```python
from build123d import *

# Parameters (mm, degrees)
SKETCH1_R           = 1.05
BOSS_EXTRUDE1_DEPTH = 1.5
FILLET1_R           = 1.5
SKETCH2_R           = 1.05
SKETCH2_W           = 4
SKETCH2_H           = 16
BOSS_EXTRUDE2_DEPTH = 1.5
SKETCH4_R           = 1.25
CUT_EXTRUDE2_DEPTH  = 160.067595694
CUT_EXTRUDE4_DEPTH  = 160.067595694
FILLET3_R           = 1
FILLET4_R           = 1.5
SKETCH6_W           = 140
SKETCH6_H           = 59.5
CUT_EXTRUDE5_DEPTH  = 10


with BuildPart() as part:
    # Sketch1 → Boss-Extrude1 (new body)
    with BuildSketch(Plane(origin=(0, 0, 0), x_dir=(0, 0, -1), z_dir=(1, 0, 0))):
        Polygon((0, 0), (0, 75.5), (21.5, 75.5), (40, 0), (35.881667859, 0), (29.755840045, 25), (4, 25), (4, 0), align=None)
        with Locations((5.5, 72.5)):
            Circle(SKETCH1_R, mode=Mode.SUBTRACT)
        with Locations((18.5, 72.5)):
            Circle(SKETCH1_R, mode=Mode.SUBTRACT)
        Polygon((4, 69.5), (18.851866535, 69.5), (4, 29), align=None, mode=Mode.SUBTRACT)
        Polygon((8.260475549, 29), (20.558388216, 62.535546651), (28.775707595, 29), align=None, mode=Mode.SUBTRACT)
    extrude(amount=BOSS_EXTRUDE1_DEPTH)

    # Fillet1
    fillet1_edges = [part.edges().sort_by_distance(p)[0] for p in [
        (0.75, 75.5, -21.5),
        (0.75, 25, -29.755840045),
        (0.75, 25, -4),
        (0.75, 69.5, -4),
        (0.75, 29, -4),
        (0.75, 69.5, -18.851866535),
        (0.75, 29, -8.260475549),
        (0.75, 29, -28.775707595),
        (0.75, 62.535546651, -20.558388216),
    ]]
    fillet(fillet1_edges, radius=FILLET1_R)

    # Sketch2 → Boss-Extrude2 (add)
    # profile 1 of 5: a face of its own
    with BuildSketch(Plane(origin=(1.5, 0, 0), x_dir=(0, 0, -1), z_dir=(1, 0, 0))):
        Polygon((70, 0), (70, 16), (36.079470199, 16), (40, 0), align=None)
    # profile 2 of 5: a face of its own
    with BuildSketch(Plane(origin=(1.5, 0, 0), x_dir=(0, 0, -1), z_dir=(1, 0, 0))):
        with BuildLine():
            Line((103.920529801, 16), (70, 16))
            Line((70, 16), (70, 0))
            Line((70, 0), (140, 0))
            Line((140, 0), (140, 16))
            Line((140, 16), (140, 75.5))
            Line((140, 75.5), (119.676824884, 75.5))
            ThreePointArc((119.676824884, 75.5), (118.750942408, 75.180144754), (118.219924421, 74.356988855))
            Line((118.219924421, 74.356988855), (103.920529801, 16))
        make_face()
        with BuildLine():
            Line((108.038861942, 16), (109.964084377, 23.856988855))
            ThreePointArc((109.964084377, 23.856988855), (110.495102363, 24.680144754), (111.420984839, 25))
            Line((111.420984839, 25), (134.5, 25))
            ThreePointArc((134.5, 25), (135.560660172, 24.560660172), (136, 23.5))
            Line((136, 23.5), (136, 16))
            Line((136, 16), (108.038861942, 16))
        make_face(mode=Mode.SUBTRACT)
        with BuildLine():
            ThreePointArc((131.000070484, 31.016439186), (130.821545012, 29.641122471), (129.591776989, 29))
            Line((129.591776989, 29), (113.136216627, 29))
            ThreePointArc((113.136216627, 29), (111.956071873, 29.574117524), (111.679316165, 30.856988855))
            Line((111.679316165, 30.856988855), (118.270545293, 57.756329353))
            ThreePointArc((118.270545293, 57.756329353), (119.644098522, 58.897023121), (121.135739251, 57.915779684))
            Line((121.135739251, 57.915779684), (131.000070484, 31.016439186))
        make_face(mode=Mode.SUBTRACT)
        with BuildLine():
            ThreePointArc((121.887587432, 67.483560814), (122.066112904, 68.858877529), (123.295880927, 69.5))
            Line((123.295880927, 69.5), (134.5, 69.5))
            ThreePointArc((134.5, 69.5), (135.560660172, 69.060660172), (136, 68))
            Line((136, 68), (136, 37.447151885))
            ThreePointArc((136, 37.447151885), (134.762259183, 35.970256452), (133.091706505, 36.930712699))
            Line((133.091706505, 36.930712699), (121.887587432, 67.483560814))
        make_face(mode=Mode.SUBTRACT)
        with Locations((121.5, 72.5)):
            Circle(SKETCH2_R, mode=Mode.SUBTRACT)
        with Locations((134.5, 72.5)):
            Circle(SKETCH2_R, mode=Mode.SUBTRACT)
    # profile 3 of 5: a face of its own
    with BuildSketch(Plane(origin=(1.5, 0, 0), x_dir=(0, 0, -1), z_dir=(1, 0, 0))):
        Polygon((35.881667859, 0), (31.961138058, 16), (4, 16), (4, 0), align=None)
    # profile 4 of 5: a face of its own
    with BuildSketch(Plane(origin=(1.5, 0, 0), x_dir=(0, 0, -1), z_dir=(1, 0, 0))):
        Polygon((40, 0), (36.079470199, 16), (31.961138058, 16), (35.881667859, 0), align=None)
    # profile 5 of 5: a face of its own
    with BuildSketch(Plane(origin=(1.5, 0, 0), x_dir=(0, 0, -1), z_dir=(1, 0, 0))):
        with Locations((2, 8)):
            Rectangle(SKETCH2_W, SKETCH2_H)
    extrude(amount=-BOSS_EXTRUDE2_DEPTH)

    # Sketch4 → Cut-Extrude2 (cut, through all)
    with BuildSketch(Plane(origin=(1.5, 0, 0), x_dir=(0, 0, -1), z_dir=(1, 0, 0))):
        with Locations((6.1, 8)):
            Circle(SKETCH4_R)
        with Locations((17.1, 8)):
            Circle(SKETCH4_R)
        with Locations(Location((122.9, 8, 0), (0, 0, 180))):
            Circle(SKETCH4_R)
        with Locations(Location((133.9, 8, 0), (0, 0, 180))):
            Circle(SKETCH4_R)
        with BuildLine():
            Line((126.4, 16), (130.4, 16))
            Line((130.4, 16), (130.4, 8))
            ThreePointArc((130.4, 8), (128.4, 6), (126.4, 8))
            Line((126.4, 8), (126.4, 16))
        make_face()
        with BuildLine():
            Line((9.6, 16), (13.6, 16))
            Line((13.6, 16), (13.6, 8))
            ThreePointArc((13.6, 8), (11.6, 6), (9.6, 8))
            Line((9.6, 8), (9.6, 16))
        make_face()
    extrude(amount=-CUT_EXTRUDE2_DEPTH, mode=Mode.SUBTRACT)

    # Sketch5 → Cut-Extrude4 (cut, through all)
    with BuildSketch(Plane(origin=(1.5, 0, 0), x_dir=(0, 0, -1), z_dir=(1, 0, 0))):
        Polygon((35.984634856, 4.5), (46, 4.5), (56.015365144, 4.5), (46, 10.342296334), align=None)
        Polygon((47.984634856, 11.5), (68.015365144, 11.5), (58, 5.657703666), align=None)
        Polygon((59.984634856, 4.5), (70, 4.5), (80.015365144, 4.5), (70, 10.342296334), align=None)
        Polygon((22, 4.5), (22, 10.342296334), (32.015365144, 4.5), align=None)
        Polygon((23.984634856, 11.5), (44.015365144, 11.5), (34, 5.657703666), align=None)
        Polygon((118, 4.5), (118, 10.342296334), (107.984634856, 4.5), align=None)
        Polygon((94, 4.5), (104.015365144, 4.5), (94, 10.342296334), (83.984634856, 4.5), align=None)
        Polygon((95.984634856, 11.5), (116.015365144, 11.5), (106, 5.657703666), align=None)
        Polygon((71.984634856, 11.5), (92.015365144, 11.5), (82, 5.657703666), align=None)
    extrude(amount=-CUT_EXTRUDE4_DEPTH, mode=Mode.SUBTRACT)

    # Fillet3
    fillet3_edges = [part.edges().sort_by_distance(p)[0] for p in [
        (0.75, 4.5, -83.984634856),
        (0.75, 4.5, -104.015365144),
        (0.75, 4.5, -80.015365144),
        (0.75, 4.5, -59.984634856),
        (0.75, 10.342296334, -70),
        (0.75, 4.5, -56.015365144),
        (0.75, 4.5, -35.984634856),
        (0.75, 10.342296334, -46),
        (0.75, 4.5, -118),
        (0.75, 4.5, -107.984634856),
        (0.75, 10.342296334, -118),
        (0.75, 11.5, -44.015365144),
        (0.75, 5.657703666, -34),
        (0.75, 11.5, -23.984634856),
        (0.75, 5.657703666, -58),
        (0.75, 11.5, -47.984634856),
        (0.75, 11.5, -68.015365144),
        (0.75, 11.5, -116.015365144),
        (0.75, 5.657703666, -106),
        (0.75, 11.5, -95.984634856),
        (0.75, 11.5, -92.015365144),
        (0.75, 5.657703666, -82),
        (0.75, 11.5, -71.984634856),
        (0.75, 4.5, -32.015365144),
        (0.75, 4.5, -22),
        (0.75, 10.342296334, -22),
    ]]
    fillet(fillet3_edges, radius=FILLET3_R)

    # Fillet4
    fillet4_edges = [part.edges().sort_by_distance(p)[0] for p in [
        (0.75, 16, -4),
        (0.75, 16, -31.961138058),
        (0.75, 16, -36.079470199),
        (0.75, 16, -136),
        (0.75, 16, -108.038861942),
        (0.75, 16, -103.920529801),
    ]]
    fillet(fillet4_edges, radius=FILLET4_R)

    # Sketch6 → Cut-Extrude5 (cut)
    with BuildSketch(Plane(origin=(1.5, 0, 0), x_dir=(0, 0, -1), z_dir=(1, 0, 0))):
        with Locations((70, 45.75)):
            Rectangle(SKETCH6_W, SKETCH6_H)
    extrude(amount=-CUT_EXTRUDE5_DEPTH, mode=Mode.SUBTRACT)


solid = part.part
```
Work out the finished part from the listing and answer in its coordinate system (mm). A direction names the side the tool comes from. Give positions to 0.01 mm unless a question says otherwise; leave off trailing zeros. Loops run counter-clockwise (first coordinate to the right, second up) from the corner with the lowest first, then second, coordinate; pieces in that order, holes last. Notation, with made-up numbers: (79, -37) -> (117, -37) arc R35 cw to (117, -1) -> close; hole circle Ø1 at (78.25, 18). An arc over 180 degrees is marked (long way). Put each result on its own line as item: value. Start each with the question number.
Item 1: The part is cut by section A-A (z = -17.1). Give the vertices of the cut face in (x, y).
Item 2: Find the intervals of material crossed by L1, parallel to Z at x = 0.75, y = 13.5; L2, parallel to Y at x = 0.3, z = -17.1; L3, parallel to Y at x = 1.2, z = -64.5, in increasing order. Write a range as [from, to].
Item 3: Which of the six approach directions +Z, -Z, +X, -X, +Y, -Y give full straight-line access (tool end or side, diameter ignored) to faces 1 (the face through (0.76, 8.23, -42.38)), 2 (the face through (0, 10, -69))?
Item 4: Each of these flat-tipped pins is pushed along its axis until it touches: P1, Ø0.8, axis at x = 0.5, z = -109, coming from the -Y side; P2, Ø2, axis at y = 8, z = -122.9, coming from the -X side (3 decimals). Where does it stop, or does it pass through?
Item 5: The part is cut by section B-B (y = 14.25). Give the vertices of the cut face in (x, z).
Item 6: The part is cut by section D-D (z = -56). Give the vertices of the cut face in (x, y).
Item 7: The part is cut by section C-C (x = 0.9). State how many separate pieces and enclosed holes the cut face has, then the cut area to 3 significant figures.
Answers below:
1. outline: (0, 0) -> (1.5, 0) -> (1.5, 6.75) -> (0, 6.75) -> close; (0, 9.25) -> (1.5, 9.25) -> (1.5, 16) -> (0, 16) -> close
2. L1: [-140, -130.4], [-126.4, -13.6], [-9.6, 0]
2. L2: [0, 6.75], [9.25, 16]
2. L3: [0, 4.5], [7.13, 9.45], [11.48, 16]
3. face 1: +X, -X
3. face 2: +Z, -Z, -X, +Y, -Y
4. P1: y = 0
4. P2: through
5. outline: (0, -140) -> (1.5, -140) -> (1.5, -130.4) -> (0, -130.4) -> close; (0, -126.4) -> (1.5, -126.4) -> (1.5, -13.6) -> (0, -13.6) -> close; (0, -9.6) -> (1.5, -9.6) -> (1.5, 0) -> (0, 0) -> close
6. outline: (0, 0) -> (1.5, 0) -> (1.5, 6.82) -> (0, 6.82) -> close; (0, 11.5) -> (1.5, 11.5) -> (1.5, 16) -> (0, 16) -> close
7. separate pieces: 1
7. enclosed holes: 13
7. area: 1,720 mm2
